Check sheet for the modelled part. Datum: model origin and axes. Units: mm. Give positions to 0.01 mm unless a question says otherwise; leave off trailing zeros. Order: outer loops, then holes, each group sorted by start corner. A loop starts at its lowest first (then second) coordinate and runs counter-clockwise, first axis right, second up.
```python
from build123d import *

# Parameters (mm, degrees)
SKETCH1_W           = 254
SKETCH1_H           = 50.8
BOSS_EXTRUDE1_DEPTH = 101.6
SKETCH2_R           = 9.525
CUT_EXTRUDE1_DEPTH  = 25.4
SKETCH3_R           = 4.7625
CUT_EXTRUDE2_DEPTH  = 25.4
SKETCH4_R           = 4.7625
CUT_EXTRUDE3_DEPTH  = 25.4
CUT_EXTRUDE4_START  = -25.4
SKETCH5_R           = 4.7625
CUT_EXTRUDE4_DEPTH  = 25.4


with BuildPart() as part:
    # Sketch1 → Boss-Extrude1 (new body)
    with BuildSketch(Plane.XY):
        Rectangle(SKETCH1_W, SKETCH1_H)
    extrude(amount=BOSS_EXTRUDE1_DEPTH)

    # Sketch2 → Cut-Extrude1 (cut)
    with BuildSketch(Plane.XY.offset(101.6)):
        with Locations((-85.598, 4.5974)):
            Circle(SKETCH2_R)
        with Locations(Location((85.598, 4.5974, 0), (0, 0, 180))):
            Circle(SKETCH2_R)
    extrude(amount=-CUT_EXTRUDE1_DEPTH, mode=Mode.SUBTRACT)

    # Sketch3 → Cut-Extrude2 (cut)
    with BuildSketch(Plane(origin=(0, 0, 0), x_dir=(-1, 0, 0), z_dir=(0, 0, -1))):
        with Locations((-57.15, 0)):
            Circle(SKETCH3_R)
        with Locations(Location((57.15, 0, 0), (0, 0, 180))):
            Circle(SKETCH3_R)
    extrude(amount=-CUT_EXTRUDE2_DEPTH, mode=Mode.SUBTRACT)

    # Sketch4 → Cut-Extrude3 (cut)
    with BuildSketch(Plane(origin=(127, 0, 0), x_dir=(0, 0, -1), z_dir=(1, 0, 0))):
        with Locations((-50.8, 0)):
            Circle(SKETCH4_R)
    extrude(amount=-CUT_EXTRUDE3_DEPTH, mode=Mode.SUBTRACT)

    # Sketch5 → Cut-Extrude4 (cut)
    with BuildSketch(Plane.ZY.offset(127).offset(CUT_EXTRUDE4_START)):
        with Locations(Location((50.8, 0, 0), (0, 0, 180))):
            Circle(SKETCH5_R)
    extrude(amount=CUT_EXTRUDE4_DEPTH, mode=Mode.SUBTRACT)


solid = part.part
```
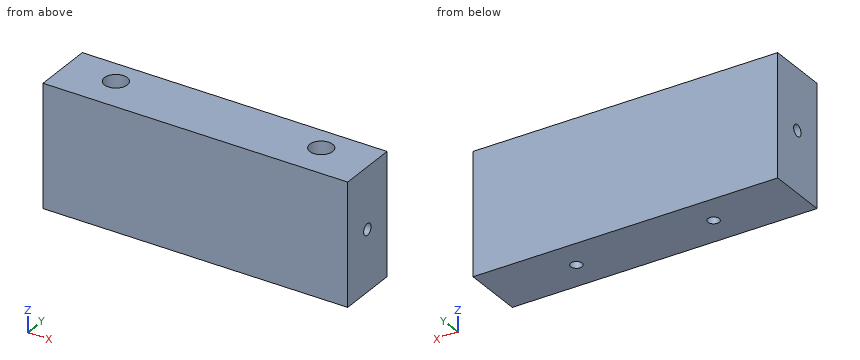
(1) Cross-section at A-A on x = -57.15. Enter the section's corners in (y, z).
Response values:
outline: (-25.4, 0) - (-4.76, 0) - (-4.76, 25.4) - (4.76, 25.4) - (4.76, 0) - (25.4, 0) - (25.4, 101.6) - (-25.4, 101.6) - close
(2) Material ranges on L1, parallel to Y at x = -57.15, z = 8.75; L2, parallel to X at y = -3, z = 9.5; L3, parallel to X at y = -4, z = 76.5, recorded low to high.
Response values:
L1: y = -25.4 to -4.76, 4.76 to 25.4
L2: x = -127 to -60.85, -53.45 to 53.45, 60.85 to 127
L3: x = -127 to -89.7, -81.5 to 81.5, 89.7 to 127
(3) Gauge pin test, flat ends, axial feed: pin 1 Ø8.5 at (x, y) = (57.15, 0) entering from -Z; pin 2 Ø5.5 at (y, z) = (0, 50.8) entering from +X. Record the tip position at first contact, or that the pin passes through.
Response values:
pin 1: stops at z = 25.4
pin 2: stops at x = 101.6
(4) Cross-section at C-C on z = 91. Enter the section's corners in (x, y) (3 decimals).
Response values:
outline: (-127, -25.4) - (127, -25.4) - (127, 25.4) - (-127, 25.4) - close; hole circle Ø19.05 at (-85.598, 4.597); hole circle Ø19.05 at (85.598, 4.597)
(5) Cross-section at D-D on y = 8. Enter the section's corners in (x, z), then the cut area to 3 significant figures.
Response values:
outline: (-127, 0) - (127, 0) - (127, 101.6) - (94.49, 101.6) - (94.49, 76.2) - (76.7, 76.2) - (76.7, 101.6) - (-76.7, 101.6) - (-76.7, 76.2) - (-94.49, 76.2) - (-94.49, 101.6) - (-127, 101.6) - close
area: 24,900 mm2
(6) Cross-section at B-B on z = 50.8. Enter the section's corners in (x, y), then the cut area to 3 significant figures.
Response values:
outline: (-127, -25.4) - (127, -25.4) - (127, -4.76) - (101.6, -4.76) - (101.6, 4.76) - (127, 4.76) - (127, 25.4) - (-127, 25.4) - (-127, 4.76) - (-101.6, 4.76) - (-101.6, -4.76) - (-127, -4.76) - close
area: 12,400 mm2
